from build123d import *

# Parameters (mm, degrees)
SKETCH1_W          = 125
SKETCH1_H          = 225
BASE_FLANGE1_DEPTH = 1.3
SKETCH6_R          = 2.25
CUT_EXTRUDE1_DEPTH = 10
FILLET1_R          = 10


# Sheet-metal steps are written as plain solids
with BuildPart() as part:
    # Sketch1 → Base-Flange1 (new body)
    with BuildSketch(Plane(origin=(0, 0, 0), x_dir=(1, 0, 0), z_dir=(0, 1, 0))):
        with Locations((-1.187869711, 9.383580575)):
            Rectangle(SKETCH1_W, SKETCH1_H)
    extrude(amount=-BASE_FLANGE1_DEPTH)

    # Sketch6 → Cut-Extrude1 (cut)
    with BuildSketch(Plane(origin=(0, 0, 0), x_dir=(1, 0, 0), z_dir=(0, 1, 0))):
        with Locations(Location((53.812130289, 114.383580575, 0), (0, 0, 270))):
            Circle(SKETCH6_R)
        with Locations(Location((53.812130289, -95.616419425, 0), (0, 0, 270))):
            Circle(SKETCH6_R)
        with Locations(Location((-56.187869711, -95.616419425, 0), (0, 0, 270))):
            Circle(SKETCH6_R)
        with Locations(Location((-56.187869711, 114.383580575, 0), (0, 0, 270))):
            Circle(SKETCH6_R)
        with Locations(Location((53.812130289, 9.383580575, 0), (0, 0, 270))):
            Circle(SKETCH6_R)
        with Locations(Location((-56.187869711, 9.383580575, 0), (0, 0, 270))):
            Circle(SKETCH6_R)
    extrude(amount=-CUT_EXTRUDE1_DEPTH, mode=Mode.SUBTRACT)

    # Fillet1
    fillet1_edges = [part.edges().sort_by_distance(p)[0] for p in [
        (61.312130289, -0.65, 103.116419425),
        (-63.687869711, -0.65, 103.116419425),
        (-63.687869711, -0.65, -121.883580575),
        (61.312130289, -0.65, -121.883580575),
    ]]
    fillet(fillet1_edges, radius=FILLET1_R)


solid = part.part
The listing builds one solid part. Answer for the finished solid, in the listing's coordinates (mm). Give positions to 0.01 mm unless a question says otherwise; leave off trailing zeros.
Item 1: Find the intervals of material crossed by line 1 along Z through (x, y) = (-58, -0.2); line 2 along Z through (x, y) = (54.5, -1.05), in increasing order.
Item 2: Determine the mould class of faces 1 (the cylindrical face through (-56.09, -0.64, -116.63)), 2 (the cylindrical face through (-60.836, -0.659, 100.109)), 3 (the flat face through (-2, 0, -11)) for opening direction Z: released by +Z, released by -Z, zero draft, split by the parting line, or undercut.
Item 3: A flat-ended cylindrical pin translates along its axis: P1, Ø5, axis at x = -56.19, z = -9.38, coming from the +Y side. Find the tip coordinate at first contact, or state that the pin passes through.
Completed:
1. line 1: z = -120.91 to -115.72, -113.05 to -10.72, -8.05 to 94.28, 96.95 to 102.14
1. line 2: z = -121.36 to -116.53, -112.24 to -11.53, -7.24 to 93.47, 97.76 to 102.59
2. face 1: undercut
2. face 2: released by +Z
2. face 3: zero draft
3. P1: stops at y = 0
